Input: part model. Units: mm. Frame: model coordinates. A direction names the side the tool comes from. Round coordinates to 2 decimals unless told otherwise and drop trailing zeros. Loops run counter-clockwise (first coordinate to the right, second up) from the corner with the lowest first, then second, coordinate; pieces in that order, holes last.
(1) Access query for faces 5 (the face through (21.804, 6.867, -2.214)), 6 (the face through (56.067, -52.343, 6.261)), 7 (the face through (-5.506, 24.796, -88.206)). Directions: +Z, -Z, +X, -X, +Y, -Y. A direction counts if a zero-diameter tool reaches every point of the face in a straight line with its end or side. Return the directions, or none.
(2) Cut plane A-A, the plane z = -24. Output: boundary loops of the cut face in (x, y) (3 decimals).
(3) Draft query along Y for faces 1 (the face through (-20, -18, 12.7)), 2 (the face through (42.397, -13.352, -46.332)), 3 (the face through (-5.506, 24.796, 5.456)), 4 (the face through (5, -16, -79.693)). Return one class per face: released by +Y, released by -Y, zero draft, split by the parting line, or undercut.
(4) First-contact query: pin 1 Ø2 at (y, z) = (-36, -17.5) entering from -X; pin 2 Ø14.5 at (x, y) = (-49.99, 49.56) entering from -Z; pin 3 Ø10 at (y, z) = (26.5, -23.5) entering from +X. Flat tips, straight axial feed; report the tip coordinate or a pass-through.
(5) Line query: line 1 (X direction, y = 0, z = -80); line 2 (Y direction, x = 0, z = 7); line 3 (X direction, y = 0, z = -84). Output: solid intervals per line, ascending.
from build123d import *

# Parameters (mm, degrees)
F0_R      = 82.55
F1_DEPTH  = 12.7
F2_R      = 44.45
F4_DEPTH  = 95.25
F3_R      = 6.35
F5_DEPTH  = 25.4
F6_R      = 15.875
F7_DEPTH  = 127
F8_R      = 25.4
F8_R_2    = 15.875
F9_DEPTH  = 14.2875
F10_R     = 15.875
F11_DEPTH = 107.951
F12_R     = 25.4
F13_DEPTH = 1.5875
F14_R     = 25.4
F14_R_2   = 15.875
F15_DEPTH = 14.2875
F16_R     = 22.86
F17_DEPTH = 1.27
F18_R     = 22.86
F19_DEPTH = 1.27
F20_SIZE  = 1.27
F21_SIZE  = 1.27


with BuildPart() as f1:
    # F0 (on Top) → F1 (new body)
    with BuildSketch(Plane.XY):
        with Locations((-0.4078939673, -0.6442572922)):
            Circle(F0_R)
    extrude(amount=F1_DEPTH)

    # F2 (on face) → F4 (join)
    with BuildSketch(Plane(origin=(0, 0, 0), x_dir=(1, 0, 0), z_dir=(0, 0, -1))):
        Circle(F2_R)
    extrude(amount=F4_DEPTH)

    # F3 (on face) → F5 (cut)
    with BuildSketch(Plane(origin=(0, 0, 0), x_dir=(1, 0, 0), z_dir=(0, 0, -1))):
        with Locations((-49.9900558808, 50.4357930472)):
            Circle(F3_R)
        with Locations((50.0097441192, -49.5640069528)):
            Circle(F3_R)
        with Locations((50.0097441192, 50.4357930472)):
            Circle(F3_R)
        with Locations((-49.9900558808, -49.5640069528)):
            Circle(F3_R)
    extrude(amount=-F5_DEPTH, mode=Mode.SUBTRACT)

    # F6 (on face) → F7 (cut)
    with BuildSketch(Plane(origin=(0, 0, 0), x_dir=(1, 0, 0), z_dir=(0, 0, -1))):
        Circle(F6_R)
    extrude(amount=F7_DEPTH, mode=Mode.SUBTRACT)

    # F8 (on face) → F9 (cut)
    with BuildSketch(Plane(origin=(0, 0, 0), x_dir=(1, 0, 0), z_dir=(0, 0, -1))):
        Circle(F8_R)
        Circle(F8_R_2, mode=Mode.SUBTRACT)
    extrude(amount=-F9_DEPTH, mode=Mode.SUBTRACT)

    # F10 (on face) → F11 (cut, through all)
    with BuildSketch(Plane(origin=(0, 0, -95.25), x_dir=(1, 0, 0), z_dir=(0, 0, -1))):
        Circle(F10_R)
    extrude(amount=-F11_DEPTH, mode=Mode.SUBTRACT)

    # F12 (on face) → F13 (cut)
    with BuildSketch(Plane.XY):
        Circle(F12_R)
    extrude(amount=-F13_DEPTH, mode=Mode.SUBTRACT)

    # F14 (on face) → F15 (cut)
    with BuildSketch(Plane(origin=(0, 0, -95.25), x_dir=(1, 0, 0), z_dir=(0, 0, -1))):
        Circle(F14_R)
        Circle(F14_R_2, mode=Mode.SUBTRACT)
    extrude(amount=-F15_DEPTH, mode=Mode.SUBTRACT)

    # F16 (on face) → F17 (cut)
    with BuildSketch(Plane(origin=(0, 0, -80.9625), x_dir=(1, 0, 0), z_dir=(0, 0, -1))):
        Circle(F16_R)
    extrude(amount=-F17_DEPTH, mode=Mode.SUBTRACT)

    # F18 (on face) → F19 (cut)
    with BuildSketch(Plane.XY.offset(-1.5875)):
        Circle(F18_R)
    extrude(amount=-F19_DEPTH, mode=Mode.SUBTRACT)

    # F20
    f20_edges = [f1.edges().sort_by_distance(p)[0] for p in [
        (-82.957894, -0.644257, 0),
    ]]
    chamfer(f20_edges, length=F20_SIZE)

    # F21
    f21_edges = [f1.edges().sort_by_distance(p)[0] for p in [
        (-44.45, 0, -95.25),
    ]]
    chamfer(f21_edges, length=F21_SIZE)


solid = f1.part
Reported:
1. face 5: +Z
1. face 6: +Z, -Z
1. face 7: -Z
2. outline: circle Ø88.9 at (0, 0); hole circle Ø31.75 at (0, 0)
3. face 1: zero draft
3. face 2: split by the parting line
3. face 3: undercut
3. face 4: undercut
4. pin 1: stops at x = -27.4
4. pin 2: stops at z = 0
4. pin 3: stops at x = 38.9
5. line 1: x = -44.45 to -22.86, 22.86 to 44.45
5. line 2: y = -83.19 to -25.4, 25.4 to 81.9
5. line 3: x = -44.45 to -25.4, 25.4 to 44.45
